For this review, take the finished solid that the model builds, in its own axes (mm). Face numbers are marked on the shaded views. A direction names the side the tool comes from. Coordinates: 2 decimals unless noted, no trailing zeros. Order: outer loops, then holes, each group sorted by start corner. A loop starts at its lowest first (then second) coordinate and runs counter-clockwise, first axis right, second up. Notation, with made-up numbers: (27, 75.25) - (86, 75.25) arc R11 cw to (86, 90.25) - close; hole circle Ø5 at (46, -28.5). An arc over 180 degrees is marked (long way). One line per item, written item: value. Start each with the question number.
(1) Consider section D-D on z = 1.1. Write out the cut boundary in (x, y), then the cut area to 3 significant figures.
(2) To check wall thickness, follow line 1 along Z through (x, y) = (-36.75, 34.5); line 2 along Z through (x, y) = (-37.5, 36.25); line 3 along X through (y, z) = (30, 0.4). State the ranges of each line that lie inside material, in increasing order.
(3) Mouldability with a two-part tool opening along X and no side actions: class the marked faces 3, 4, 5 and 6 as released by +X, released by -X, zero draft, split by the parting line, or undercut.
(4) Consider section B-B on y = 33.25. Write out the cut boundary in (x, z) (3 decimals), then the cut area to 3 significant figures.
(5) Consider section A-A on x = -33.75. Write out the cut boundary in (y, z).
(6) For the marked faces 1 and 2, list the 3-axis set-ups (+Z, -Z, +X, -X, +Y, -Y) from which the entire face can be reached by the end or side of a thin tool; tool diameter is ignored.
(7) Consider section C-C on z = 0.5. Write out the cut boundary in (x, y), then the cut area to 3 significant figures.
```python
from build123d import *

# Parameters (mm, degrees)
F0_W        = 7.62
F0_H        = 7.62
F1_DEPTH    = 1.27
F2_T1_DEPTH = 13.97
F3_W        = 5.1244873625
F3_H        = 0.6355810037
F4_DEPTH    = 7.62


# Not quite as in the source:
# - a fillet or chamfer that OpenCascade refuses, or shapes differently, is made with other operations: its cross-section is extruded or revolved along the edge and cut away or added


with BuildPart() as f1:
    # F0 (on Top) → F1 (new body)
    with BuildSketch(Plane.XY):
        with Locations((-34.8768493396, 33.171152453)):
            Rectangle(F0_W, F0_H)
    extrude(amount=F1_DEPTH)

    # F2: fillet of radius 1.27 on 4 edges, made by hand

    # F2_s2 → F2_t1 (cut)
    with BuildSketch(Plane.XZ.offset(-40.156152453)):
        with BuildLine():
            ThreePointArc((-38.6868493396, 0), (-38.3148749517, 0.8980256121), (-37.4168493396, 1.27))
            Line((-37.4168493396, 1.27), (-38.6868493396, 1.27))
            Line((-38.6868493396, 1.27), (-38.6868493396, 0))
        make_face()
        with BuildLine():
            ThreePointArc((-31.0668493396, 0), (-31.4388237275, 0.8980256121), (-32.3368493396, 1.27))
            Line((-32.3368493396, 1.27), (-31.0668493396, 1.27))
            Line((-31.0668493396, 1.27), (-31.0668493396, 0))
        make_face()
        with BuildLine():
            ThreePointArc((-38.6868493396, 1.27), (-38.3148749517, 0.3719743879), (-37.4168493396, 0))
            Line((-37.4168493396, 0), (-38.6868493396, 0))
            Line((-38.6868493396, 0), (-38.6868493396, 1.27))
        make_face()
        with BuildLine():
            ThreePointArc((-31.0668493396, 1.27), (-31.4388237275, 0.3719743879), (-32.3368493396, 0))
            Line((-32.3368493396, 0), (-31.0668493396, 0))
            Line((-31.0668493396, 0), (-31.0668493396, 1.27))
        make_face()
    extrude(amount=F2_T1_DEPTH, mode=Mode.SUBTRACT)

    # F3 (on face) → F4 (cut)
    with BuildSketch(Plane(origin=(0, 36.981152453, 0), x_dir=(-1, 0, 0), z_dir=(0, 1, 0))):
        with Locations((34.8990930209, 0.6385907036)):
            Rectangle(F3_W, F3_H)
    extrude(amount=-F4_DEPTH, mode=Mode.SUBTRACT)


solid = f1.part
```
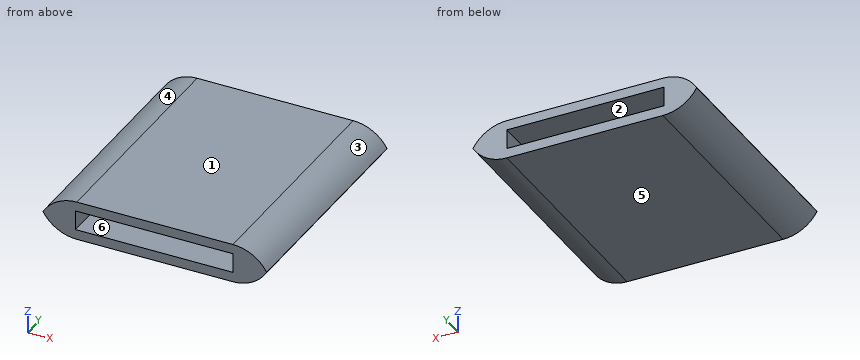
Geometry check:
1. outline: (-38.05, 29.36) - (-31.7, 29.36) - (-31.7, 36.98) - (-38.05, 36.98) - close
1. area: 48.4 mm^2
2. line 1: z = 0 to 0.32, 0.96 to 1.27
2. line 2: z = 0 to 1.27
2. line 3: x = -38.34 to -37.46, -32.34 to -31.41
3. face 3: released by +X
3. face 4: released by -X
3. face 5: zero draft
3. face 6: undercut
4. outline: (-38.517, 0.635) arc R1.27 ccw to (-37.417, 0) - (-32.337, 0) arc R1.27 ccw to (-31.237, 0.635) arc R1.27 ccw to (-32.337, 1.27) - (-37.417, 1.27) arc R1.27 ccw to start; hole (-37.461, 0.321) - (-32.337, 0.321) - (-32.337, 0.956) - (-37.461, 0.956) - close
4. area: 5.18 mm^2
5. outline: (29.36, 0) - (36.98, 0) - (36.98, 0.32) - (29.36, 0.32) - close; (29.36, 0.96) - (36.98, 0.96) - (36.98, 1.27) - (29.36, 1.27) - close
6. face 1: +Z, +X, -X, +Y, -Y
6. face 2: +Y, -Y
7. outline: (-38.43, 29.36) - (-37.46, 29.36) - (-37.46, 36.98) - (-38.43, 36.98) - close; (-32.34, 29.36) - (-31.33, 29.36) - (-31.33, 36.98) - (-32.34, 36.98) - close
7. area: 15.1 mm^2
